Check sheet for the drawn part. Datum: minimum x, y, z corner. Units: mm. A direction names the side the tool comes from. Coordinates: 2 decimals unless noted, no trailing zeros. Write each loop counter-clockwise with the first axis right and the second up, starting at its lowest first coordinate (ties: lowest second). Pieces come first, ordered by that corner, then holes. Notation, with made-up numbers: (-30.75, -16) -> (13.25, -16) arc R21 ccw to (13.25, 5) -> close; hole circle Ø8 at (-20, 80.5). An arc over 180 degrees is marked (long way). Answer in a Markdown table with one row per item. Add a question column.
Q1. Section check B-B, the plane z = 20.5. Record the boundary of the cut face in (x, y), and give its area (3 significant figures).
Q2. Section check C-C, the plane y = 13. Record the boundary of the cut face in (x, z), and give its area (3 significant figures).
Q3. Thickness scan on line 1 (X direction, y = 13, z = 29.4); line 2 (Y direction, x = 22.5, z = 28.4); line 3 (X direction, y = 15, z = 20). Record the ranges inside material, lowest first.
Q4. Gauge pin test, flat ends, axial feed: P1, Ø2, axis at x = 7.5, y = 13, coming from the +Z side; P2, Ø8, axis at x = 26.5, y = 9, coming from the -Z side. Record the tip position at first contact, or that the pin passes through.
Q5. Section check D-D, the plane y = 9.5. Record the boundary of the cut face in (x, z).
Q6. Section check A-A, the plane x = 7.5. Record the boundary of the cut face in (y, z).
Q7. Release check for a two-part mould opening along X. For the marked faces 3, 4 and 5 record: pulls with the +X half, pulls with the -X half, needs draft (parallel to the pull), parting line crosses it, or undercut.
Q8. Tool access check on the marked faces 1 and 2. Record the directions out of +Z, -Z, +X, -X, +Y, -Y that give a thin tool (end or side, any length) a straight path to the whole face; none if there is none.
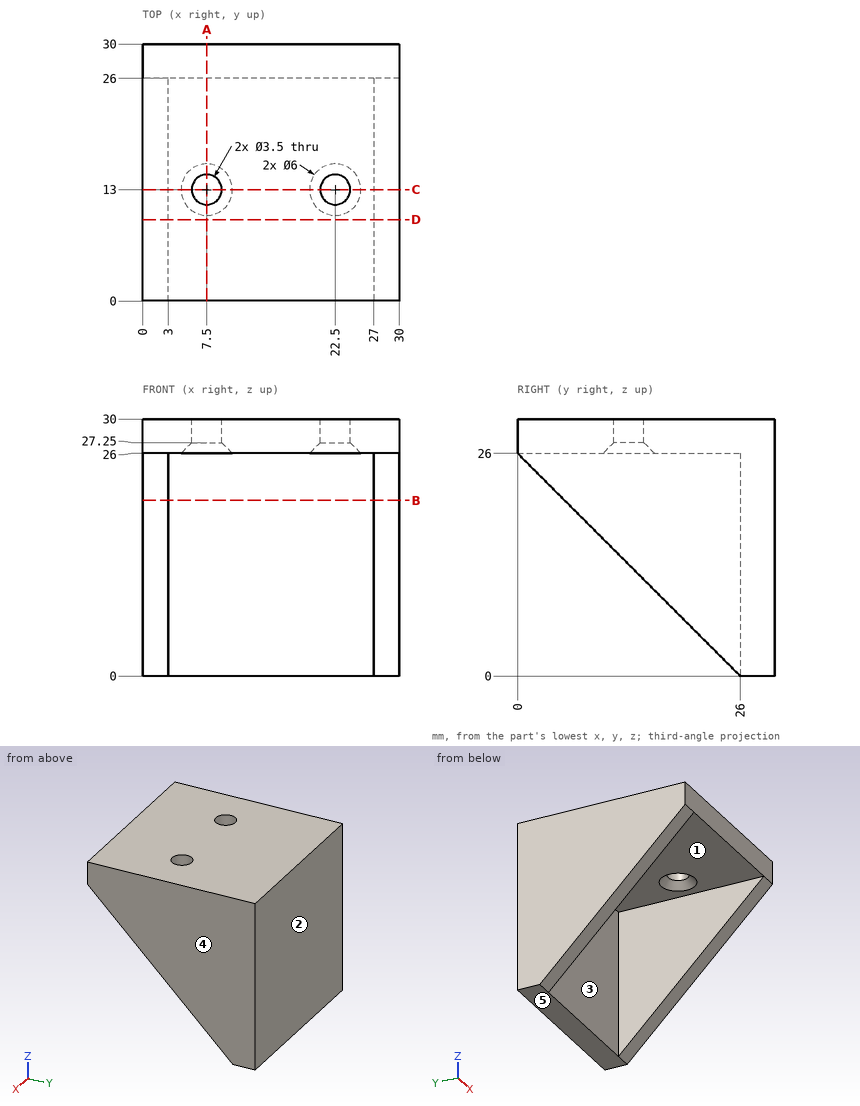
Calculated:
| question | item | result |
|---|---|---|
| 1 | outline | (0, 5.5) -> (3, 5.5) -> (3, 26) -> (27, 26) -> (27, 5.5) -> (30, 5.5) -> (30, 30) -> (0, 30) -> close |
| 1 | area | 243 mm² |
| 2 | outline | (0, 13) -> (3, 13) -> (3, 26) -> (4.5, 26) -> (5.75, 27.25) -> (5.75, 30) -> (0, 30) -> close; (9.25, 27.25) -> (10.5, 26) -> (19.5, 26) -> (20.75, 27.25) -> (20.75, 30) -> (9.25, 30) -> close; (24.25, 27.25) -> (25.5, 26) -> (27, 26) -> (27, 13) -> (30, 13) -> (30, 30) -> (24.25, 30) -> close |
| 2 | area | 167 mm² |
| 3 | line 1 | x = 0 to 5.75, 9.25 to 20.75, 24.25 to 30 |
| 3 | line 2 | y = 0 to 11.25, 14.75 to 30 |
| 3 | line 3 | x = 0 to 3, 27 to 30 |
| 4 | P1 | passes through |
| 4 | P2 | stops at z = 13.03 |
| 5 | outline | (0, 16.5) -> (3, 16.5) -> (3, 26) -> (27, 26) -> (27, 16.5) -> (30, 16.5) -> (30, 30) -> (0, 30) -> close |
| 6 | outline | (0, 26) -> (10, 26) -> (11.25, 27.25) -> (11.25, 30) -> (0, 30) -> close; (14.75, 27.25) -> (16, 26) -> (26, 26) -> (26, 0) -> (30, 0) -> (30, 30) -> (14.75, 30) -> close |
| 7 | face 3 | undercut |
| 7 | face 4 | pulls with the +X half |
| 7 | face 5 | needs draft |
| 8 | face 1 | -Z, -Y |
| 8 | face 2 | +Z, -Z, +X, -X, +Y |
